Here's the drawing with two shaded views (mm, measured from the low corner). I have some questions. A direction names the side the tool comes from. Coordinates: 2 decimals unless noted, no trailing zeros. Write each loop counter-clockwise with the first axis right and the second up, starting at its lowest first coordinate (ties: lowest second). Pieces come first, ordered by that corner, then holes.
Item 1: I want a section at C-C on y = 9.25. Please give me the cut outline in (x, z).
Item 2: Thinking about a two-plate mould opening in Y: for the marked faces 3, 4, 5 and 6, which applies, +Y half, -Y half, draft (parallel to the pull), parting line (faces both ways), or undercut?
Item 3: I want a section at A-A on x = 14.75. Please give me the cut outline in (y, z).
Item 4: If I drill on probe 1 along Y at (x, z) = (17, 1); probe 2 along Y at (x, z) = (20, 2); probe 3 along X at (y, z) = (9.75, 11), over which ranges is the centre line in solid material (lowest first)?
Item 5: Which directions (+Z, -Z, +X, -X, +Y, -Y) give clear straight access to the entire face, cutting with the end or side of a thin tool? Please do the marked faces 1 and 2.
Item 6: For P1, Ø8, axis at x = 5.5, z = 10.5, coming from the +Y side; P2, Ø2, axis at y = 14.5, z = 9.5, coming from the -X side; P3, Ø6, axis at y = 16, z = 15, coming from the -X side, each with a flat end and sliding along its axis, tell me the tip position at first contact or that it passes through.
Item 7: I want a section at D-D on x = 7.25. Please give me the cut outline in (y, z).
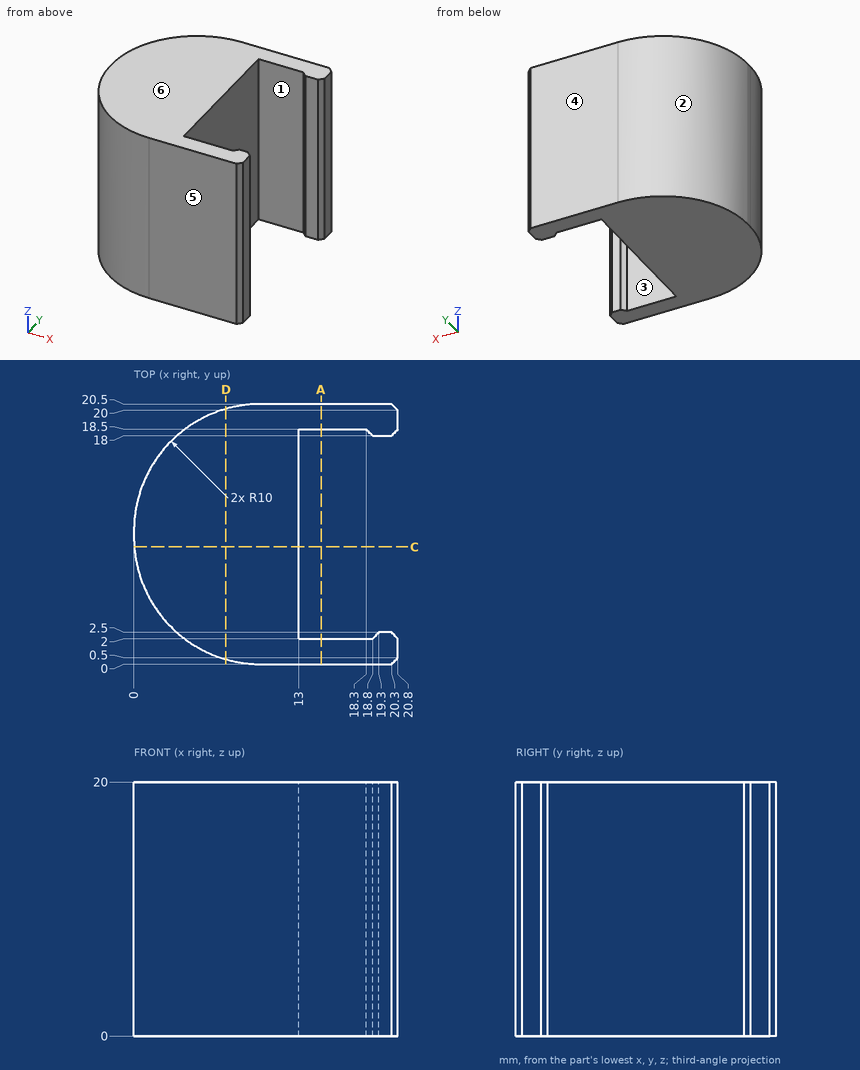
Response values:
1. outline: (0.03, 0) - (13, 0) - (13, 20) - (0.03, 20) - close
2. face 3: undercut
2. face 4: +Y half
2. face 5: -Y half
2. face 6: draft
3. outline: (0, 0) - (2, 0) - (2, 20) - (0, 20) - close; (18.5, 0) - (20.5, 0) - (20.5, 20) - (18.5, 20) - close
4. probe 1: y = 0 to 2, 18.5 to 20.5
4. probe 2: y = 0 to 2.5, 18 to 20.5
4. probe 3: x = 0 to 13
5. face 1: +Z, -Z
5. face 2: +Z, -Z, -X, +Y
6. P1: stops at y = 20.49
6. P2: stops at x = 0.46
6. P3: stops at x = 0.32
7. outline: (0.39, 0) - (20.11, 0) - (20.11, 20) - (0.39, 20) - close
